```python
from build123d import *

# Parameters (mm, degrees)
SKETCH1_W           = 320
SKETCH1_H           = 20
BOSS_EXTRUDE1_DEPTH = 10
SKETCH2_R           = 2.5
BOSS_EXTRUDE2_DEPTH = 10
SKETCH4_R           = 6
CUT_EXTRUDE1_DEPTH  = 60
SKETCH5_W           = 280
SKETCH5_H           = 10
BOSS_EXTRUDE3_DEPTH = 20
SKETCH6_R           = 5.912914271
CUT_EXTRUDE2_DEPTH  = 20


with BuildPart() as part:
    # Sketch1 → Boss-Extrude1 (new body)
    with BuildSketch(Plane.XY):
        with Locations((-160, 10)):
            Rectangle(SKETCH1_W, SKETCH1_H)
    extrude(amount=BOSS_EXTRUDE1_DEPTH)

    # Sketch2 → Boss-Extrude2 (add)
    with BuildSketch(Plane.XY.offset(10)):
        with Locations((-10, 10)):
            Circle(SKETCH2_R)
    boss_extrude2 = extrude(amount=BOSS_EXTRUDE2_DEPTH)

    # Mirror1: Boss-Extrude2 across plane
    add(boss_extrude2.mirror(Plane(origin=(-160, 0, 0), x_dir=(0, 0, 1), z_dir=(1, 0, 0))))

    # Sketch4 → Cut-Extrude1 (cut)
    with BuildSketch(Plane.XY.offset(10)):
        with Locations((-160, 10)):
            Circle(SKETCH4_R)
    extrude(amount=-CUT_EXTRUDE1_DEPTH, mode=Mode.SUBTRACT)

    # Sketch5 → Boss-Extrude3 (add)
    with BuildSketch(Plane(origin=(0, 20, 0), x_dir=(1, 0, 0), z_dir=(0, 1, 0))):
        with Locations((-160, -5)):
            Rectangle(SKETCH5_W, SKETCH5_H)
    extrude(amount=BOSS_EXTRUDE3_DEPTH)

    # Sketch6 → Cut-Extrude2 (cut)
    with BuildSketch(Plane(origin=(0, 0, 0), x_dir=(-1, 0, 0), z_dir=(0, 0, -1))):
        with Locations((237.401391361, 23.777250692)):
            Circle(SKETCH6_R)
    cut_extrude2 = extrude(amount=-CUT_EXTRUDE2_DEPTH, mode=Mode.SUBTRACT)

    # Mirror2: Cut-Extrude2 across plane
    add(cut_extrude2.mirror(Plane(origin=(-160, 0, 0), x_dir=(0, 0, 1), z_dir=(1, 0, 0))), mode=Mode.SUBTRACT)


solid = part.part
```
Part model, mm, in its own coordinate system. A direction names the side the tool comes from. Coordinates: 2 decimals unless noted, no trailing zeros. Loops run counter-clockwise (first coordinate to the right, second up) from the corner with the lowest first, then second, coordinate; pieces in that order, holes last. Notation, with made-up numbers: (76, 38) - (119, 38) arc R17 cw to (119, 42) - close; hole circle Ø3 at (2, 34.25). An arc over 180 degrees is marked (long way). Write item = value, one per line. Start each with the question number.
Item 1: 3-axis set-ups, long thin cutter, end or side, ignore diameter. For faces 4 (the flat face through (-300, 30, 5)), 5 (the flat face through (-20, 30, 5)), 6 (the cylindrical face through (-312.31, 9.04, 14.93)), 7 (the cylindrical face through (-243.041, 25.553, 4.93)), 8 (the flat face through (-162, 40, 5)): which of +Z, -Z, +X, -X, +Y, -Y reach the whole face in a straight line?
Item 2: Cut at C-C, the plane x = -52.5. Give the cut face in (y, z).
Item 3: Cut at A-A, the plane x = -160. Give the cut face in (y, z), and give its area (3 significant figures).
Item 4: Cut at B-B, the plane z = 12.75. Give the cut face in (x, y).
Item 5: Wall check: L1, parallel to Y at x = -83, z = 6.5; L2, parallel to X at y = 19, z = 6.5; L3, parallel to Z at x = -102, y = 15. Give the ranges that are in metal, low to high. Write a range as from..to.
Item 6: Flat gauge pins, fed straight in: pin 1 Ø1 at (x, y) = (-88.5, 22.5) entering from -Z; pin 2 Ø5 at (x, z) = (-314, 6.5) entering from +Y; pin 3 Ø3 at (y, z) = (31.5, 5.5) entering from +X; pin 4 Ø8 at (x, y) = (-172.5, 34) entering from +Z. Where does each tip first touch, or does it go through?
Item 7: Mould opens along Y. For faces 1 (the cylindrical face through (-10.54, 7.56, 14.93)), 2 (the cylindrical face through (-164.76, 6.35, 5.07)), 3 (the flat face through (-10, 20, 5)) say: released by +Y, released by -Y, zero draft, split by the parting line, or undercut.
The answers:
q1.face_4 = +Z, -Z, -X, +Y
q1.face_5 = +Z, -Z, +X, +Y
q1.face_6 = +Z
q1.face_7 = +Z, -Z
q1.face_8 = +Z, -Z, +X, -X, +Y
q2.outline = (0, 0) - (40, 0) - (40, 10) - (0, 10) - close
q3.outline = (0, 0) - (4, 0) - (4, 10) - (0, 10) - close; (16, 0) - (40, 0) - (40, 10) - (16, 10) - close
q3.area = 280 mm2
q4.outline = circle Ø5 at (-310, 10); circle Ø5 at (-10, 10)
q5.L1 = 0..17.88, 29.68..40
q5.L2 = -320..-240.89, -233.92..-86.08, -79.11..0
q5.L3 = 0..10
q6.pin_1 = 0
q6.pin_2 = 20
q6.pin_3 = -20
q6.pin_4 = 10
q7.face_1 = split by the parting line
q7.face_2 = undercut
q7.face_3 = released by +Y
